from build123d import *

# Parameters (mm, degrees)
ESQUISSE1_R             = 32
ESQUISSE1_R_2           = 17
BOSS_EXTRU_1_DEPTH      = 15
ESQUISSE1_R_3           = 19
ESQUISSE1_R_4           = 10
BOSS_EXTRU_1_2_DEPTH    = 15
BOSS_EXTRU_2_DEPTH      = 5
ESQUISSE3_R             = 27.5
ESQUISSE3_R_2           = 21.5
ENL_V_MAT_EXTRU_1_DEPTH = 5
ESQUISSE4_R             = 21.5
ESQUISSE4_R_2           = 17
BOSS_EXTRU_3_DEPTH      = 7.5


with BuildPart() as part:
    # Esquisse1 → Boss.-Extru.1 (new body, symmetric)
    with BuildSketch(Plane.XY):
        Circle(ESQUISSE1_R)
        Circle(ESQUISSE1_R_2, mode=Mode.SUBTRACT)
    extrude(amount=BOSS_EXTRU_1_DEPTH, both=True)



with BuildPart() as body_2:
    # Esquisse1 → Boss.-Extru.1 2 (new body, symmetric)
    with BuildSketch(Plane.XY):
        with Locations((0, 75)):
            Circle(ESQUISSE1_R_3)
        with Locations((0, 75)):
            Circle(ESQUISSE1_R_4, mode=Mode.SUBTRACT)
    extrude(amount=BOSS_EXTRU_1_2_DEPTH, both=True)


with BuildPart() as part_1:
    add(part.part)

    add(body_2.part)  # Boss.-Extru.2 merges body 2
    # Esquisse2 → Boss.-Extru.2 (add, symmetric)
    with BuildSketch(Plane.XY):
        with BuildLine():
            ThreePointArc((26.678302647, 17.671111111), (0, 32), (-26.678302647, 17.671111111))
            ThreePointArc((-26.678302647, 17.671111111), (-16.836772686, 42.914041255), (-18.321243986, 69.966907631))
            ThreePointArc((-18.321243986, 69.966907631), (0, 56), (18.321243986, 69.966907631))
            ThreePointArc((18.321243986, 69.966907631), (16.836772686, 42.914041255), (26.678302647, 17.671111111))
        make_face()
    extrude(amount=BOSS_EXTRU_2_DEPTH, both=True)

    # Esquisse3 → Enlèv. mat.-Extru.1 (cut)
    with BuildSketch(Plane(origin=(0, 0, -15), x_dir=(-1, 0, 0), z_dir=(0, 0, -1))):
        Circle(ESQUISSE3_R)
        Circle(ESQUISSE3_R_2, mode=Mode.SUBTRACT)
    extrude(amount=-ENL_V_MAT_EXTRU_1_DEPTH, mode=Mode.SUBTRACT)

    # Esquisse4 → Boss.-Extru.3 (add, symmetric)
    with BuildSketch(Plane(origin=(0, 0, -15), x_dir=(-1, 0, 0), z_dir=(0, 0, -1))):
        Circle(ESQUISSE4_R)
        Circle(ESQUISSE4_R_2, mode=Mode.SUBTRACT)
    extrude(amount=BOSS_EXTRU_3_DEPTH, both=True)


solid = part_1.part
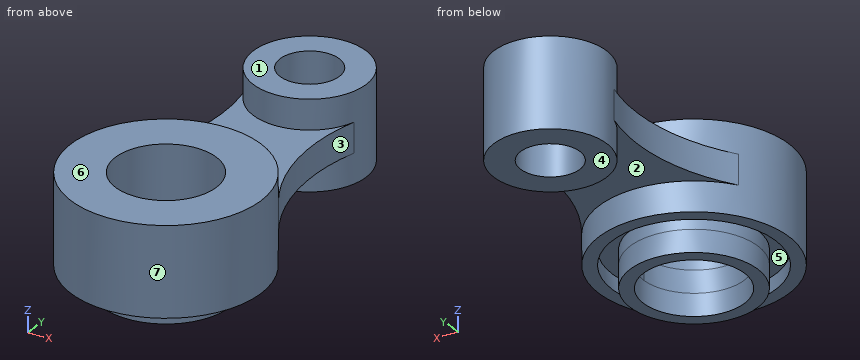
Here's how the part is built. I have some questions about the finished solid (model axes, mm). Face numbers are marked on the shaded views. A direction names the side the tool comes from. Round coordinates to 2 decimals unless told otherwise and drop trailing zeros. Write each loop counter-clockwise with the first axis right and the second up, starting at its lowest first coordinate (ties: lowest second). Pieces come first, ordered by that corner, then holes. Notation, with made-up numbers: (88.5, 26) -> (131.5, 26) arc R8 cw to (131.5, 34) -> close; hole circle Ø10 at (21, 60.25). An arc over 180 degrees is marked (long way). One line per item, written item: value.
1) Suppose I cut it at D-D on x = 14.5. List the corners of the cut face in (y, z) for me.
Filled sheet:
outline: (-28.53, -15) -> (-23.37, -15) -> (-23.37, -10) -> (-15.87, -10) -> (-15.87, -22.5) -> (-8.87, -22.5) -> (-8.87, 15) -> (-28.53, 15) -> close; (8.87, -22.5) -> (15.87, -22.5) -> (15.87, -10) -> (23.37, -10) -> (23.37, -15) -> (28.53, -15) -> (28.53, -5) -> (62.72, -5) -> (62.72, -15) -> (87.28, -15) -> (87.28, 15) -> (62.72, 15) -> (62.72, 5) -> (28.53, 5) -> (28.53, 15) -> (8.87, 15) -> close
2) Suppose I cut it at C-C on y = -9.5. List the corners of the cut face in (x, z) for me, plus the area to 3 significant figures.
Filled sheet:
outline: (-30.56, -15) -> (-25.81, -15) -> (-25.81, -10) -> (-19.29, -10) -> (-19.29, -22.5) -> (-14.1, -22.5) -> (-14.1, 15) -> (-30.56, 15) -> close; (14.1, -22.5) -> (19.29, -22.5) -> (19.29, -10) -> (25.81, -10) -> (25.81, -15) -> (30.56, -15) -> (30.56, 15) -> (14.1, 15) -> close
area: 1,000 mm2
3) We'd pull the mould along Y, two halves only. Please class the marked faces 1 and 2: released by +Y, released by -Y, zero draft, split by the parting line, or undercut.
Filled sheet:
face 1: zero draft
face 2: undercut
4) If I drill on line 1 (Y direction, x = 0, z = -1.75); line 2 (Y direction, x = 0, z = -13); line 3 (Y direction, x = -15, z = 5.5), over which ranges is the centre line in solid material (lowest first)? Write a range as [from, to].
Filled sheet:
line 1: y = [-32, -17], [17, 65], [85, 94]
line 2: y = [-32, -27.5], [-21.5, -17], [17, 21.5], [27.5, 32], [56, 65], [85, 94]
line 3: y = [-28.27, -8], [8, 28.27], [63.34, 86.66]
5) For the marked faces 3, 4, 5, 6 and 7, which set-ups out of +Z, -Z, +X, -X, +Y, -Y let a thin tool reach every point of the face, with its end or its side?
Filled sheet:
face 3: +Z, -Z, +X
face 4: -Z, +X, -X, +Y
face 5: -Z
face 6: +Z, +X, -X, +Y, -Y
face 7: none
6) Suppose I cut it at B-B on z = -12. List the corners of the cut face in (x, y) for me, plus the area to 3 significant figures.
Filled sheet:
outline: circle Ø64 at (0, 0); circle Ø43 at (0, 0); circle Ø38 at (0, 75); hole circle Ø55 at (0, 0); hole circle Ø34 at (0, 0); hole circle Ø20 at (0, 75)
area: 2,210 mm2
7) Suppose I cut it at A-A on x = 0. List the corners of the cut face in (y, z) for me.
Filled sheet:
outline: (-32, -15) -> (-27.5, -15) -> (-27.5, -10) -> (-21.5, -10) -> (-21.5, -22.5) -> (-17, -22.5) -> (-17, 15) -> (-32, 15) -> close; (17, -22.5) -> (21.5, -22.5) -> (21.5, -10) -> (27.5, -10) -> (27.5, -15) -> (32, -15) -> (32, -5) -> (56, -5) -> (56, -15) -> (65, -15) -> (65, 15) -> (56, 15) -> (56, 5) -> (32, 5) -> (32, 15) -> (17, 15) -> close; (85, -15) -> (94, -15) -> (94, 15) -> (85, 15) -> close
8) I'm going to push flat-ended pins straight in: pin 1 Ø16 at (x, y) = (0, 75) entering from -Z; pin 2 Ø2 at (x, z) = (-4, 8.5) entering from -Y; pin 3 Ø3 at (x, y) = (13.5, 44.5) entering from +Z; pin 4 Ø1.5 at (y, z) = (-16.5, -2.5) entering from +X. Where does each tip first touch, or does it pass through?
Filled sheet:
pin 1: passes through
pin 2: stops at y = -31.86
pin 3: stops at z = 5
pin 4: stops at x = 27.86
